For this review, use the dimensioned drawing (mm, ordinates from the lowest corner) and the shaded views. Give positions to 0.01 mm unless a question says otherwise; leave off trailing zeros. Loops run counter-clockwise (first coordinate to the right, second up) from the corner with the lowest first, then second, coordinate; pieces in that order, holes last. Notation, with made-up numbers: (27, 51.25) -> (75, 51.25) arc R28 cw to (75, 83.25) -> close; hole circle Ø11 at (39, -13.75). An arc over 180 degrees is marked (long way). Write each question's results on one line, items separated by ' | '. Start each with the question number.
Q1. We need section A-A (x = 150). Write out the cut boundary in (y, z).
Q2. Mouldability with a two-part tool opening along Y and no side actions: class the marked faces 1, 2 and 3 as released by +Y, released by -Y, zero draft, split by the parting line, or undercut.
Q3. Insertion check: pin 1 Ø3 at (x, y) = (149.5, 21) entering from -Z. The pin has a flat end and moves straight along its axis. Give the tip position at first contact, or say it passes through.
Q4. Wall thickness on L1, parallel to Y at x = 150, z = 67; L2, parallel to X at y = 31, z = 57.5; L3, parallel to Y at x = 157.5, z = 48.5: over which ranges is each line inside the solid? List them lowest first. Write a range as [from, to].
Q5. We need section B-B (y = 50). Write out the cut boundary in (x, z).
Q6. We need section C-C (z = 132). Write out the cut boundary in (x, y).
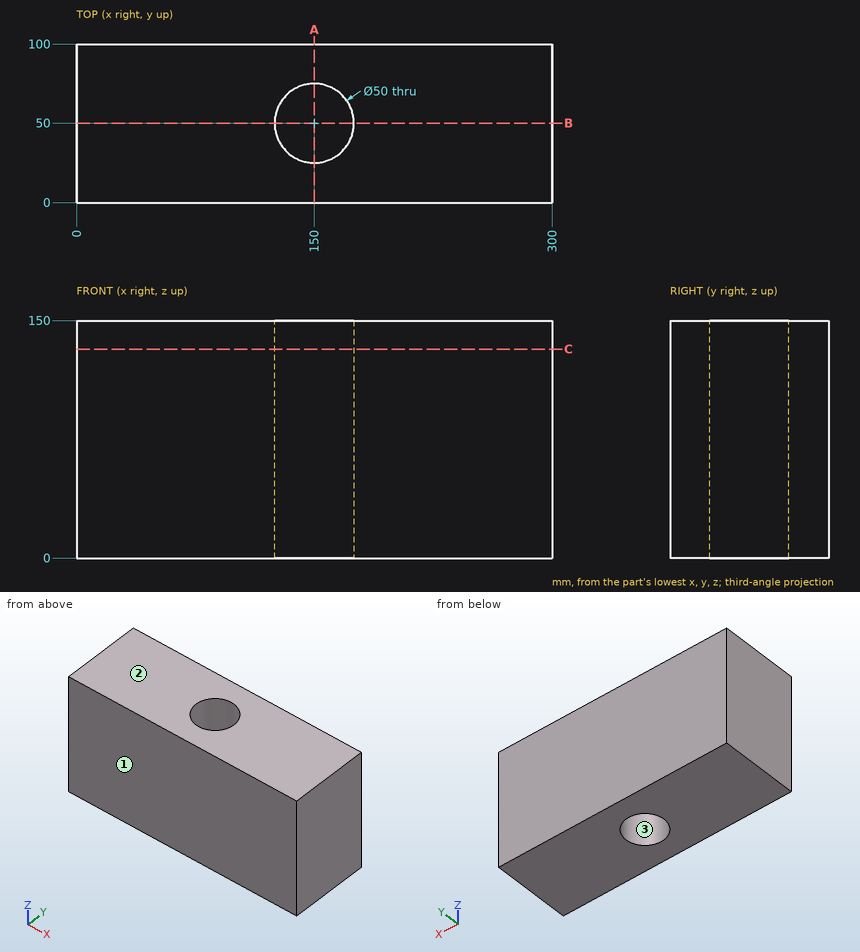
Output:
1) outline: (0, 0) -> (25, 0) -> (25, 150) -> (0, 150) -> close; (75, 0) -> (100, 0) -> (100, 150) -> (75, 150) -> close
2) face 1: released by -Y | face 2: zero draft | face 3: undercut
3) pin 1: z = 0
4) L1: [0, 25], [75, 100] | L2: [0, 133.75], [166.25, 300] | L3: [0, 26.15], [73.85, 100]
5) outline: (0, 0) -> (125, 0) -> (125, 150) -> (0, 150) -> close; (175, 0) -> (300, 0) -> (300, 150) -> (175, 150) -> close
6) outline: (0, 0) -> (300, 0) -> (300, 100) -> (0, 100) -> close; hole circle Ø50 at (150, 50)
